from build123d import *

# Parameters (mm, degrees)
F0_W     = 100
F0_H     = 100
F1_DEPTH = 45
F6_DEPTH = 15


with BuildPart() as f1:
    # F0 (on Top) → F1 (new body)
    with BuildSketch(Plane.XY):
        Rectangle(F0_W, F0_H)
    extrude(amount=F1_DEPTH)

    # F5 (on offset) → F6 (cut)
    with BuildSketch(Plane.XY.offset(45)):
        Polygon((50, -7.071068), (50, 7.071068), (-7.071068, -50), (7.071068, -50), align=None)
        Polygon((7.071068, 50), (-7.071068, 50), (-50, 7.071068), (-50, -7.071068), align=None)
    extrude(amount=-F6_DEPTH, mode=Mode.SUBTRACT)

    # F3 (on offset) → F7 section 0
    with BuildSketch(Plane.XY.offset(30)):
        Polygon((14.142136, -50), (50, -14.142136), (50, 14.142136), (-14.142136, -50), align=None)
    # F5 (on offset) → F7 section 1
    with BuildSketch(Plane.XY.offset(45)):
        Polygon((50, -7.071068), (50, 7.071068), (-7.071068, -50), (7.071068, -50), align=None)
    loft(mode=Mode.SUBTRACT)

    # F3 (on offset) → F8 section 0
    with BuildSketch(Plane.XY.offset(30)):
        Polygon((-50, -14.142136), (14.142136, 50), (-14.142136, 50), (-50, 14.142136), align=None)
    # F5 (on offset) → F8 section 1
    with BuildSketch(Plane.XY.offset(45)):
        Polygon((7.071068, 50), (-7.071068, 50), (-50, 7.071068), (-50, -7.071068), align=None)
    loft(mode=Mode.SUBTRACT)


solid = f1.part
Geometry: final body of the model. Coordinates: model frame, mm. Give positions to 0.01 mm unless a question says otherwise; leave off trailing zeros. Answer in a Markdown table with one row per item.
(1) Section query A-A on z = 40.5. State how many separate pieces and enclosed holes the cut face has, then the cut area to 3 significant figures.
Answers below:
| item | result |
|---|---|
| separate pieces | 3 |
| enclosed holes | 0 |
| area | 8,160 mm^2 |
(2) Ray query, line 1 along Y through (x, z) = (-35, 32); line 2 along Z through (x, y) = (27, -29); line 3 along Y through (x, z) = (42, 32.5). Return the intervals inside material, ascending. Write a range as [from, to].
Answers below:
| item | result |
|---|---|
| line 1 | [-50, 1.8], [28.2, 50] |
| line 2 | [0, 30] |
| line 3 | [-50, -20.96], [4.96, 50] |
(3) Draft query along X for faces 1 (the flat face through (23, -22, 30)), 2 (the flat face through (-50, -1, 22)), 3 (the flat face through (-26, 25, 30)), 4 (the flat face through (-1, 1, 45)). Return one class per face: +X half, -X half, draft (parallel to the pull), parting line (faces both ways), or undercut.
Answers below:
| item | result |
|---|---|
| face 1 | undercut |
| face 2 | -X half |
| face 3 | undercut |
| face 4 | draft |
